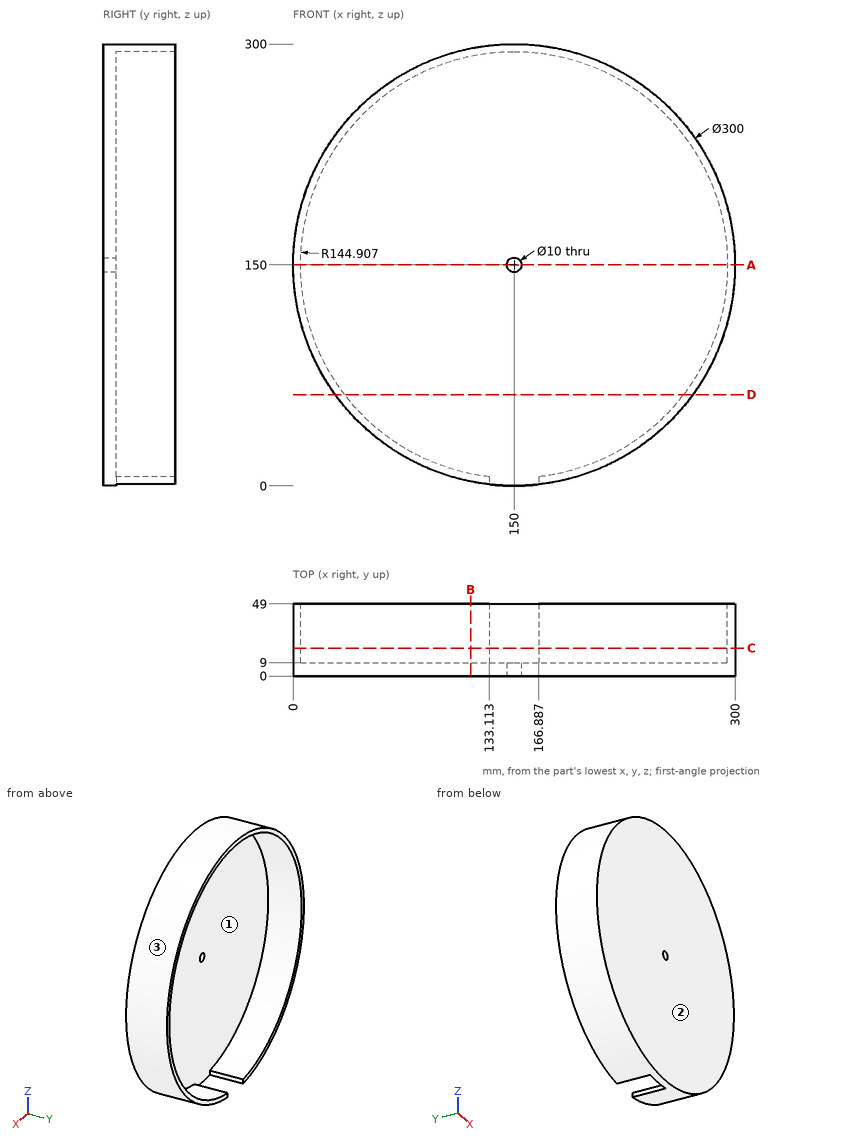
The figure shows three views and two pictorial views of one solid part (mm, origin at its lowest corner). Answer the questions. Round coordinates to 2 decimals unless told otherwise and drop trailing zeros. Order: outer loops, then holes, each group sorted by start corner. A loop starts at its lowest first (then second) coordinate and runs counter-clockwise, first axis right, second up. Notation, with made-up numbers: M 2,-28.5 L 26,-28.5 A35 cw 26,7.5 Z; hole C 21.25,34.25 d9. An arc over 180 degrees is marked long. Put each result on its own line as item: value. Start each with the question number.
Q1. Section C-C, the plane y = 19 is taken. Write down the section's boundary in (x, z), and give its area (3 significant figures).
Q2. Straight lines are drawn through the part: L1, parallel to X at y = 5, z = 150; L2, parallel to X at y = 18, z = 60.5; L3, parallel to Y at x = 126, z = 262.5. For each, find the intervals that lie inside material, in ascending order. Write a range as [from, to].
Q3. Section D-D, the plane z = 62 is taken. Write down the section's boundary in (x, y), and give its area (3 significant figures).
Q4. Section B-B, the plane x = 120.5 is taken. Write down the section's boundary in (y, z), and give its area (3 significant figures).
Q5. For a pull along Z with two mould halves and no side action, classify the marked faces 1, 2 and 3 as pulls with the +Z half, pulls with the -Z half, needs draft (parallel to the pull), parting line crosses it, or undercut.
Q6. Section A-A, the plane z = 150 is taken. Write down the section's boundary in (x, y).
Q7. Flat-ended cylindrical pins translate along their axes: pin 1 (11.5 mm diameter, centred on x = 150, z = 150, fed in from +Y); pin 2 (8 mm diameter, centred on x = 228.5, y = 35, fed in from -Z); pin 3 (10 mm diameter, centred on y = 14, z = 72.5, fed in from +X). Find the tip coordinate at first contact, or state that the pin passes through.
Findings below:
1. outline: M 133.11,0.95 L 133.11,6.08 A144.91 cw long 166.89,6.08 L 166.89,0.95 A150 ccw long Z
1. area: 4,550 mm^2
2. L1: x = [0, 145], [155, 300]
2. L2: x = [29.63, 36.04], [263.96, 270.37]
2. L3: y = [0, 9]
3. outline: M 28.53,0 L 271.47,0 L 271.47,49 L 265.13,49 L 265.13,9 L 34.87,9 L 34.87,49 L 28.53,49 Z
3. area: 2,690 mm^2
4. outline: M 0,2.93 L 49,2.93 L 49,8.13 L 9,8.13 L 9,291.87 L 49,291.87 L 49,297.07 L 0,297.07 Z
4. area: 3,060 mm^2
5. face 1: undercut
5. face 2: needs draft
5. face 3: parting line crosses it
6. outline: M 0,0 L 145,0 L 145,9 L 5.09,9 L 5.09,49 L 0,49 Z; M 155,0 L 300,0 L 300,49 L 294.91,49 L 294.91,9 L 155,9 Z
7. pin 1: stops at y = 9
7. pin 2: stops at z = 19.81
7. pin 3: stops at x = 281.32
